from build123d import *

# Parameters (mm, degrees)
SKETCH_1_W                  = 80
SKETCH_1_H                  = 80
SKETCH_1_W_2                = 40.4
SKETCH_1_H_2                = 40.4
EXTRUDE_273_DEPTH           = 8
EXTRUDE_START               = -10
EXTRUDE_351_DEPTH           = 20
CUT_EXTRUDE_442_DEPTH       = 197.214168703
CUT_EXTRUDE_442_DEPTH_BACK  = 197.214168703
CUT_EXTRUDE_500_DEPTH       = 197.214168703
CUT_EXTRUDE_500_DEPTH_BACK  = 197.214168703
SKETCH_4_R                  = 9
CUT_EXTRUDE_M4_DEPTH        = 197.214168703
CUT_EXTRUDE_M4_DEPTH_BACK   = 197.214168703
SKETCH_5_R                  = 2.25
CUT_EXTRUDE_M4_2_DEPTH      = 197.214168703
CUT_EXTRUDE_M4_2_DEPTH_BACK = 197.214168703
SKETCH_6_R                  = 2.25


with BuildPart() as part:
    # 草图1 → Extrude 273 (new body)
    with BuildSketch(Plane(origin=(0, 0, 0), x_dir=(1, 0, 0), z_dir=(0, 1, 0))):
        Rectangle(SKETCH_1_W, SKETCH_1_H)
        Rectangle(SKETCH_1_W_2, SKETCH_1_H_2, mode=Mode.SUBTRACT)
    extrude(amount=EXTRUDE_273_DEPTH)

    # 草图2 → Extrude 351 (add)
    with BuildSketch(Plane.XY.offset(EXTRUDE_START)):
        Polygon((-30, 8), (25, 8), (140, 80), (150, 80), (150, 120), (-30, 120), align=None)
    extrude(amount=EXTRUDE_351_DEPTH)

    # 草图3 → Cut-Extrude 442 (cut, two sides: drawn at the far end of the back side and taken through both)
    with BuildSketch(Plane.XY.offset(-CUT_EXTRUDE_442_DEPTH_BACK)):
        Polygon((25, 30), (100, 80), (25, 80), align=None)
    extrude(amount=CUT_EXTRUDE_442_DEPTH + CUT_EXTRUDE_442_DEPTH_BACK, mode=Mode.SUBTRACT)

    # 草图4 → Cut-Extrude 500 (cut, two sides: drawn at the far end of the back side and taken through both)
    with BuildSketch(Plane.XY.offset(-CUT_EXTRUDE_500_DEPTH_BACK)):
        with Locations((60, 100)):
            Circle(SKETCH_4_R)
        with Locations((90, 100)):
            Circle(SKETCH_4_R)
    extrude(amount=CUT_EXTRUDE_500_DEPTH + CUT_EXTRUDE_500_DEPTH_BACK, mode=Mode.SUBTRACT)

    # 草图5 → Cut-Extrude M4 (cut, two sides: drawn at the far end of the back side and taken through both)
    with BuildSketch(Plane.XY.offset(-CUT_EXTRUDE_M4_DEPTH_BACK)):
        with Locations((125, 90)):
            Circle(SKETCH_5_R)
        with Locations((125, 110)):
            Circle(SKETCH_5_R)
    extrude(amount=CUT_EXTRUDE_M4_DEPTH + CUT_EXTRUDE_M4_DEPTH_BACK, mode=Mode.SUBTRACT)

    # 草图6 → Cut-Extrude M4 2 (cut, two sides: drawn at the far end of the back side and taken through both)
    with BuildSketch(Plane(origin=(0, 0, 0), x_dir=(1, 0, 0), z_dir=(0, 1, 0)).offset(-CUT_EXTRUDE_M4_2_DEPTH_BACK)):
        with Locations(Location((-32, -32, 0), (0, 0, 270))):
            Circle(SKETCH_6_R)
        with Locations(Location((-32, 32, 0), (0, 0, 270))):
            Circle(SKETCH_6_R)
        with Locations(Location((32, -32, 0), (0, 0, 270))):
            Circle(SKETCH_6_R)
        with Locations(Location((32, 32, 0), (0, 0, 270))):
            Circle(SKETCH_6_R)
    extrude(amount=CUT_EXTRUDE_M4_2_DEPTH + CUT_EXTRUDE_M4_2_DEPTH_BACK, mode=Mode.SUBTRACT)


solid = part.part
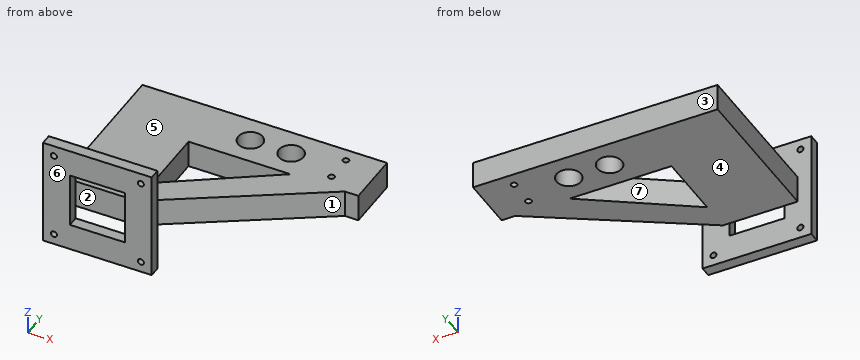
Input: part model. Units: mm. Frame: model coordinates. Face numbers are marked on the shaded views. A direction names the side the tool comes from. Round coordinates to 2 decimals unless told otherwise and drop trailing zeros. Write each loop counter-clockwise with the first axis right and the second up, starting at its lowest first coordinate (ties: lowest second). Pieces come first, ordered by that corner, then holes.
1) Draft query along X for the marked faces 1, 2 and 3. Return one class per face: pulls with the +X half, pulls with the -X half, needs draft (parallel to the pull), parting line crosses it, or undercut.
2) Ray query, L1, parallel to X at y = 100, z = -1; L2, parallel to Z at x = -32, y = 2. Return the intervals inside material, ascending.
3) Cut plane D-D (y = 65.5). Return the cut outline in (x, z), then the cut area to 3 significant figures.
4) Cut plane B-B (z = -32). Return the cut outline in (x, y), then the cut area to 3 significant figures.
5) Cut plane A-A (x = 0.5). Return the cut outline in (y, z).
6) Contact query for flat-ended pins moving along their axis: P1, Ø10, axis at x = 63, z = -1, coming from the -Y side; P2, Ø2, axis at y = 21.5, z = -9.5, coming from the -X side; P3, Ø3, axis at x = 143, z = 0.5, coming from the -Y side; P4, Ø3.5, axis at x = 125, y = 90, coming from the +Z side. Output: stop coordinate, or through.
7) Reachability of the marked faces 4, 5, 6 and 7 from +Z, -Z, +X, -X, +Y, -Y: full face, straight path, thin tool, end or side. Return the list, or none.
8) Cut plane C-C (x = 32). Return the cut outline in (y, z), then the cut area to 3 significant figures.
Geometry says:
1. face 1: pulls with the +X half
1. face 2: undercut
1. face 3: needs draft
2. L1: x = -30 to 51, 69 to 81, 99 to 150
2. L2: z = -40 to -34.25, -29.75 to 29.75, 34.25 to 40
3. outline: (-30, -10) - (25, -10) - (25, 10) - (-30, 10) - close; (78.25, -10) - (116.84, -10) - (116.84, 10) - (78.25, 10) - close
3. area: 1,870 mm2
4. outline: (-40, 0) - (-34.25, 0) - (-34.25, 8) - (-40, 8) - close; (-29.75, 0) - (29.75, 0) - (29.75, 8) - (-29.75, 8) - close; (34.25, 0) - (40, 0) - (40, 8) - (34.25, 8) - close
4. area: 568 mm2
5. outline: (0, -40) - (8, -40) - (8, -20.2) - (0, -20.2) - close; (0, 20.2) - (8, 20.2) - (8, 40) - (0, 40) - close; (8, -10) - (120, -10) - (120, 10) - (8, 10) - close
6. P1: stops at y = 28.66
6. P2: stops at x = -30
6. P3: stops at y = 80
6. P4: passes through
7. face 4: -Z, +X, -X, +Y
7. face 5: +Z, +X, -X, +Y
7. face 6: +Z, -Z, +X, -X, -Y
7. face 7: +Z, -Z
8. outline: (0, -40) - (8, -40) - (8, -34.25) - (0, -34.25) - close; (0, -29.75) - (8, -29.75) - (8, 29.75) - (0, 29.75) - close; (0, 34.25) - (8, 34.25) - (8, 40) - (0, 40) - close; (12.38, -10) - (34.67, -10) - (34.67, 10) - (12.38, 10) - close; (80, -10) - (120, -10) - (120, 10) - (80, 10) - close
8. area: 1,810 mm2
